Could you check a few things on this drawing? It's one solid part, dimensions in mm from its lowest x, y, z. A direction names the side the tool comes from. Give positions to 0.01 mm unless a question says otherwise; leave off trailing zeros. Write each loop counter-clockwise with the first axis right and the second up, starting at its lowest first coordinate (ties: lowest second). Pieces come first, ordered by that corner, then holes.
1. I'm going to push flat-ended pins straight in: pin 1 (6 mm diameter, centred on x = 23.5, y = 32, fed in from +Z); pin 2 (3 mm diameter, centred on y = 3.5, z = 3.5, fed in from -X); pin 3 (1.2 mm diameter, centred on x = 39.5, z = 3.5, fed in from +Y); pin 4 (3 mm diameter, centred on x = 3, z = 3.5, fed in from -Y). Where does each tip first touch, or does it pass through?
2. Suppose I cut it at A-A (z = 3.4). Please give me the cut outline in (x, y), and give its area (3 significant figures).
3. If I drill on probe 1 along Y at (x, z) = (21.5, 0.3); probe 2 along X at (y, z) = (38, 0.3), over which ranges is the centre line in solid material (lowest first)?
4. On a 3-axis mill with a long thin cutter (end or side, diameter ignored), from which of +Z, -Z, +X, -X, +Y, -Y can I reach the whole of each face in a straight line? I mean the marked faces 1, 2, 3, 4 and 5. Say none if no direction works.
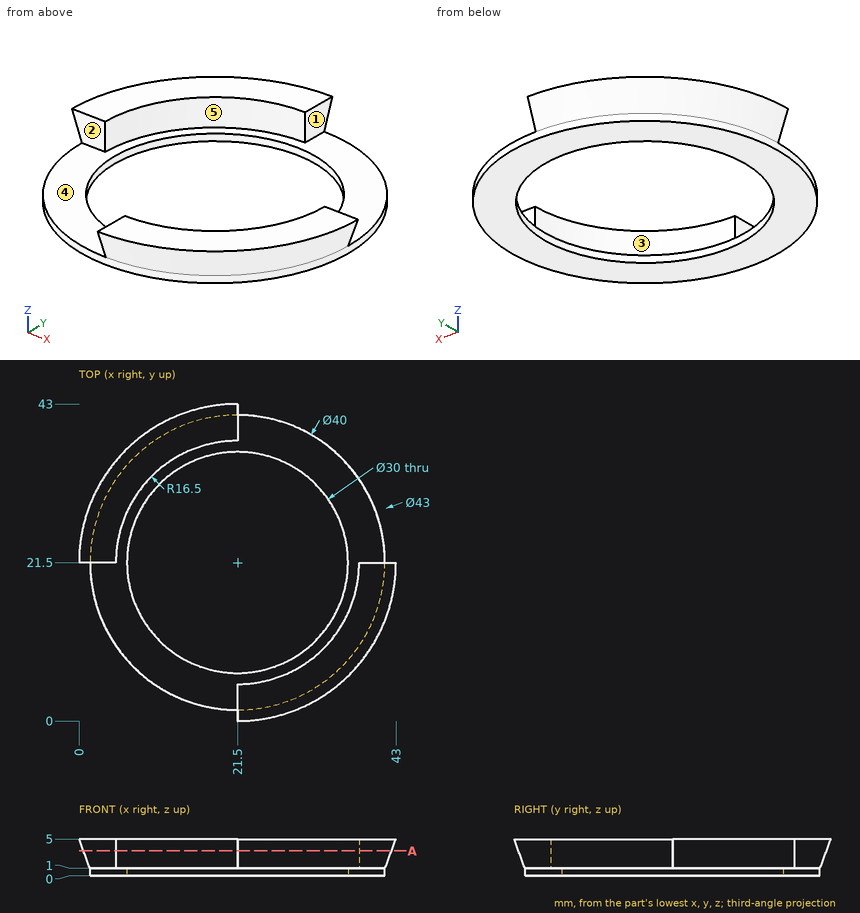
Checks:
1. pin 1: passes through
1. pin 2: stops at x = 21.5
1. pin 3: stops at y = 21.5
1. pin 4: stops at y = 21.5
2. outline: (0.6, 21.5) - (5, 21.5) arc R16.5 cw to (21.5, 38) - (21.5, 42.4) arc R20.9 ccw to start; (21.5, 0.6) arc R20.9 ccw to (42.4, 21.5) - (38, 21.5) arc R16.5 cw to (21.5, 5) - close
2. area: 258 mm2
3. probe 1: y = 1.5 to 6.5, 36.5 to 41.5
3. probe 2: x = 10.2 to 32.8
4. face 1: +Z, +X, +Y
4. face 2: +Z, -X, -Y
4. face 3: +Z, -X, +Y
4. face 4: +Z
4. face 5: +Z, +X, -Y
